Check sheet for the modelled part. Datum: model origin and axes. Units: mm. A direction names the side the tool comes from. Round coordinates to 2 decimals unless told otherwise and drop trailing zeros. Loops run counter-clockwise (first coordinate to the right, second up) from the corner with the lowest first, then second, coordinate; pieces in that order, holes last. Notation, with made-up numbers: M 66,16 L 91,16 A18 cw 91,40 Z; hole C -38.5,78.25 d10. An arc over 180 degrees is marked long. One line per question, with ' | ' between items. Start each with the question number.
(1) Section check C-C (z = 6). Record the boundary of the cut face in (x, y).
(2) Tool access check on faces 1 (the face through (8, 8, -24)), 2 (the face through (-13.887, 10.648, -11.832)), 3 (the face through (-1, -17, 3)). Record the directions out of +Z, -Z, +X, -X, +Y, -Y that give a thin tool (end or side, any length) a straight path to the whole face; none if there is none.
(3) Draft check along X on faces 4 (the face through (-5.598, 42.634, 6.902)), 5 (the face through (-8.67, -39.05, 7.68)), 6 (the face through (-1.68, 7.743, -19.204)), 7 (the face through (19, 1, 0)). Enter one of: +X half, -X half, draft (parallel to the pull), parting line (faces both ways), or undercut.
(4) Section check B-B (z = -11). Record the boundary of the cut face in (x, y), and give its area (3 significant figures).
(5) Go/stop test with flat-tipped pins: P1, Ø1.5, axis at y = -21.5, z = 7.5, coming from the +X side; P2, Ø18, axis at x = 0, y = 0.18, coming from the -Z side; P3, Ø5, axis at x = -3.5, y = -21, coming from the -Z side. Record where each tip stops, or that it passes through.
(6) Thickness scan on probe 1 along Y at (x, z) = (0, -6); probe 2 along Y at (x, z) = (0, 7); probe 3 along X at (y, z) = (0, -14.65). Record the ranges inside material, lowest first. Write a range as [from, to].
```python
from build123d import *

# Parameters (mm, degrees)
SKETCH_R        = 43
PAD_DEPTH       = 3
SKETCH001_R     = 43
SKETCH001_R_2   = 40
PAD001_DEPTH    = 11
SKETCH002_R     = 12.4
POCKET_DEPTH    = 5
SKETCH003_R     = 17.5
SKETCH003_R_2   = 12.4
PAD002_DEPTH    = 13
SKETCH004_R     = 17.5
SKETCH004_R_2   = 6
PAD003_DEPTH    = 3
SKETCH005_R     = 17.5
SKETCH005_R_2   = 7.75
PAD004_DEPTH    = 8
CHAMFER_SIZE    = 1.5
CHAMFER001_SIZE = 1.5
CHAMFER002_SIZE = 1.5


with BuildPart() as part:
    # Sketch → Pad (new body)
    with BuildSketch(Plane.XY):
        Circle(SKETCH_R)
    extrude(amount=PAD_DEPTH)

    # Sketch001 (on Face3 of Pad) → Pad001 (join)
    with BuildSketch(Plane.XY.offset(3)):
        Circle(SKETCH001_R)
        Circle(SKETCH001_R_2, mode=Mode.SUBTRACT)
    extrude(amount=PAD001_DEPTH)

    # Sketch002 (on Face6 of Pad001) → Pocket (cut)
    with BuildSketch(Plane.XY.offset(3)):
        Circle(SKETCH002_R)
    extrude(amount=-POCKET_DEPTH, mode=Mode.SUBTRACT)

    # Sketch003 (on Face2 of Pocket) → Pad002 (join)
    with BuildSketch(Plane(origin=(0, 0, 0), x_dir=(1, 0, 0), z_dir=(0, 0, -1))):
        Circle(SKETCH003_R)
        Circle(SKETCH003_R_2, mode=Mode.SUBTRACT)
    extrude(amount=PAD002_DEPTH)

    # Sketch004 (on Face6 of Pad002) → Pad003 (join)
    with BuildSketch(Plane(origin=(0, 0, -13), x_dir=(1, 0, 0), z_dir=(0, 0, -1))):
        Circle(SKETCH004_R)
        Circle(SKETCH004_R_2, mode=Mode.SUBTRACT)
    extrude(amount=PAD003_DEPTH)

    # Sketch005 (on Face8 of Pad003) → Pad004 (join)
    with BuildSketch(Plane(origin=(0, 0, -16), x_dir=(1, 0, 0), z_dir=(0, 0, -1))):
        Circle(SKETCH005_R)
        with Locations((0, -0.177664)):
            Circle(SKETCH005_R_2, mode=Mode.SUBTRACT)
    extrude(amount=PAD004_DEPTH)

    # Chamfer
    chamfer_edges = [part.edges().sort_by_distance(p)[0] for p in [
        (-7.75, 0.177664, -24),
    ]]
    chamfer(chamfer_edges, length=CHAMFER_SIZE)

    # Chamfer001
    chamfer001_edges = [part.edges().sort_by_distance(p)[0] for p in [
        (-40, 0, 14),
    ]]
    chamfer(chamfer001_edges, length=CHAMFER001_SIZE)

    # Chamfer002
    chamfer002_edges = [part.edges().sort_by_distance(p)[0] for p in [
        (-12.4, 0, 3),
    ]]
    chamfer(chamfer002_edges, length=CHAMFER002_SIZE)


solid = part.part
```
The answers:
1) outline: C 0,0 d86; hole C 0,0 d80
2) face 1: -Z, +X, -X, +Y, -Y | face 2: -Z | face 3: +Z
3) face 4: parting line | face 5: undercut | face 6: undercut | face 7: draft
4) outline: C 0,0 d35; hole C 0,0 d24.8 | area: 479 mm²
5) P1: x = 37.66 | P2: z = -23.75 | P3: z = 0
6) probe 1: [-17.5, -12.4], [12.4, 17.5] | probe 2: [-43, -40], [40, 43] | probe 3: [-17.5, -6], [6, 17.5]
